from build123d import *

# Parameters (mm, degrees)
SKETCH1_W                   = 65.087862113
SKETCH1_H                   = 182.149999994
BOSS_EXTRUDE1_DEPTH         = 6.35
F_1_4_0_25_DIAMETER_HOLE1_D = 6.35
HOLE1_D                     = 3.175
HOLE1_DEPTH                 = 31.75
HOLE1_CSINK_D               = 10.16
HOLE1_CSINK_ANGLE           = 82
HOLE1_TIP                   = 0.953866233


with BuildPart() as part:
    # Sketch1 → Boss-Extrude1 (new body)
    with BuildSketch(Plane.XY):
        with Locations((-267.296898237, -72.024999997)):
            Rectangle(SKETCH1_W, SKETCH1_H)
    extrude(amount=BOSS_EXTRUDE1_DEPTH)

    # 1/4 (0.25) Diameter Hole1 (through all)
    with Locations(Plane.XY.offset(6.35)):
        with Locations((-259.576391655, -72.024999997)):
            Hole(F_1_4_0_25_DIAMETER_HOLE1_D / 2)

    # Hole1
    with Locations(Plane(origin=(181.039434513, -72.024999997, 6.35), x_dir=(0, 1, 0), z_dir=(0, 0, 1))):
        with Locations((81.549999997, 448.336332751), (-81.549999997, 448.336332751)):
            CounterSinkHole(HOLE1_D / 2, HOLE1_CSINK_D / 2, depth=HOLE1_DEPTH, counter_sink_angle=HOLE1_CSINK_ANGLE)
            with Locations((0, 0, -(HOLE1_DEPTH + HOLE1_TIP / 2))):  # 118° drill point
                Cone(0, HOLE1_D / 2, HOLE1_TIP, mode=Mode.SUBTRACT)


solid = part.part
Source: CAD feature listing. Evaluate the final solid. Frame: model axes, mm. Coordinates: 2 decimals unless noted, no trailing zeros. One line per question, with ' | ' between items.
1) Pull-direction query (Y, two-part tool) for faces 1 (the face through (-268, -163.1, 3)), 2 (the face through (-265.58, -153.19, 2.53)), 3 (the face through (-268, -71, 0)); classes: released by +Y, released by -Y, zero draft, split by the parting line, or undercut.
Report:
face 1: released by -Y | face 2: undercut | face 3: zero draft
2) First-contact query: P1, Ø2.5, axis at x = -267.3, y = -153.57, coming from the -Z side; P2, Ø1, axis at x = -267, y = -71, coming from the -Z side. Flat tips, straight axial feed; report the tip coordinate or a pass-through.
Report:
P1: passes through | P2: stops at z = 0
3) Line query: line 1 along Y through (x, z) = (-260, 4); line 2 along Y through (x, z) = (-259, 3.25). Output: solid intervals per line, ascending.
Report:
line 1: y = -163.1 to -75.17, -68.88 to 19.05 | line 2: y = -163.1 to -75.15, -68.9 to 19.05
